Can you work these out from the model? Positions are in its coordinate system, mm. Face numbers are marked on the shaded views. A direction names the side the tool comes from. Round coordinates to 2 decimals unless told otherwise and drop trailing zeros. Order: outer loops, then holes, each group sorted by start corner. A loop starts at its lowest first (then second) coordinate and runs counter-clockwise, first axis right, second up. Notation, with made-up numbers: M 37.5,-9.5 L 62.5,-9.5 A14 cw 62.5,1.5 Z; hole C 81,-36 d1. An arc over 180 degrees is marked long. Answer as a JSON object with one key per item and string values. Group by question number.
from build123d import *

# Parameters (mm, degrees)
BASE_EXTRUSION_DEPTH    = 11
ESQUISSE2_R             = 4
ENL_V_MAT_EXTRU_1_DEPTH = 79.487260113
CHANFREIN1_SIZE         = 0.5
ESQUISSE3_R             = 4
ENL_V_MAT_EXTRU_3_DEPTH = 76.099025835
CHANFREIN2_SIZE         = 0.5
ESQUISSE4_R             = 2
ENL_V_MAT_EXTRU_4_DEPTH = 21.849235277


with BuildPart() as part:
    # Esquisse1 → Base-Extrusion (new body)
    with BuildSketch(Plane.XY):
        with BuildLine():
            Line((23.059250232, 31.5), (52.331191161, 31.5))
            Line((52.331191161, 31.5), (63, 20.831191161))
            Line((63, 20.831191161), (63, 16.5))
            Line((63, 16.5), (25, 16.5))
            Line((25, 16.5), (25, 8.5))
            Line((25, 8.5), (23.059250232, 8.5))
            ThreePointArc((23.059250232, 8.5), (11.332267447, 10.043886573), (0.40445916, 14.570332972))
            Line((0.40445916, 14.570332972), (-15.998711306, 24.040707856))
            ThreePointArc((-15.998711306, 24.040707856), (-20.208003449, 39.75), (-4.498711306, 43.959292144))
            Line((-4.498711306, 43.959292144), (11.90445916, 34.488917259))
            ThreePointArc((11.90445916, 34.488917259), (17.285105485, 32.260180577), (23.059250232, 31.5))
        make_face()
    extrude(amount=BASE_EXTRUSION_DEPTH)

    # Esquisse2 → Enlèv. mat.-Extru.1 (cut, through all)
    with BuildSketch(Plane.XY.offset(11)):
        with Locations((-10.248711306, 34)):
            Circle(ESQUISSE2_R)
    extrude(amount=-ENL_V_MAT_EXTRU_1_DEPTH, mode=Mode.SUBTRACT)

    # Chanfrein1
    chanfrein1_edges = [part.edges().sort_by_distance(p)[0] for p in [
        (-14.248711306, 34, 0),
        (-14.248711306, 34, 11),
    ]]
    chamfer(chanfrein1_edges, length=CHANFREIN1_SIZE)

    # Esquisse3 → Enlèv. mat.-Extru.3 (cut, through all)
    with BuildSketch(Plane(origin=(23.483322458, -13.431543362, 11), x_dir=(1, 0, 0), z_dir=(0, 0, 1))):
        with Locations((-9.483322458, 33.431543362)):
            Circle(ESQUISSE3_R)
    extrude(amount=-ENL_V_MAT_EXTRU_3_DEPTH, mode=Mode.SUBTRACT)

    # Chanfrein2
    chanfrein2_edges = [part.edges().sort_by_distance(p)[0] for p in [
        (10, 20, 0),
        (10, 20, 11),
    ]]
    chamfer(chanfrein2_edges, length=CHANFREIN2_SIZE)

    # Esquisse4 → Enlèv. mat.-Extru.4 (cut)
    with BuildSketch(Plane.XZ.offset(-16.5)):
        with Locations(Location((35, 5.5, 0), (0, 0, 270))):
            Circle(ESQUISSE4_R)
        with Locations(Location((53, 5.5, 0), (0, 0, 270))):
            Circle(ESQUISSE4_R)
    extrude(amount=-ENL_V_MAT_EXTRU_4_DEPTH, mode=Mode.SUBTRACT)


solid = part.part
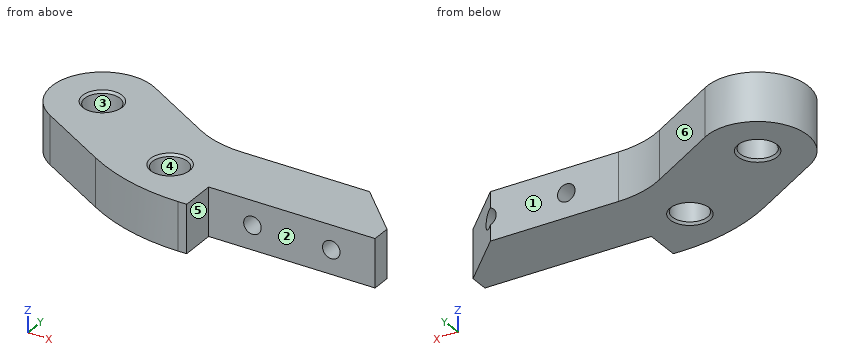
Item 1: Suppose I cut it at C-C, the plane z = 5.5. Write out the boundary of the cut face in (x, y), and give its area (3 significant figures).
Item 2: I need wall thicknesses on line 1 (X direction, y = 18, z = 5.5); line 2 (X direction, y = 21.5, z = 8.25); line 3 (X direction, y = 22.75, z = 5.5). Which ranges of each line are inside material? Lowest first, please.
Item 3: If we mould it in two halves opening along Y, with no side actions, what happens to the marked faces 4, 5 and 6? For each: +Y half, -Y half, draft (parallel to the pull), parting line (faces both ways), or undercut.
Item 4: Suppose I cut it at B-B, the plane x = 35. Write out the boundary of the cut face in (y, z), and give its area (3 significant figures).
Item 5: Suppose I cut it at A-A, the plane y = 20. Write out the boundary of the cut face in (x, z).
Item 6: Suppose I cut it at D-D, the plane z = 1.75. Write out the boundary of the cut face in (x, y), and give its area (3 significant figures).
Item 7: I'm going to push flat-ended pins straight in: pin 1 Ø1.5 at (x, z) = (-8.5, 4.5) entering from -Y; pin 2 Ø5.5 at (x, z) = (38, 5.5) entering from +Y; pin 3 Ø5.5 at (x, z) = (40.5, 3) entering from -Y. Where does each tip first touch, or does it pass through?
Item 8: On a 3-axis mill with a long thin cutter (end or side, diameter ignored), from which of +Z, -Z, +X, -X, +Y, -Y can I reach the whole of each face in a straight line? I mean the marked faces 1, 2 and 3. Say none if no direction works.
Computed:
{
 "1": {"outline": "M -16,24.04 L 0.4,14.57 A45.31 ccw 23.06,8.5 L 25,8.5 L 25,16.5 L 33,16.5 L 33,31.5 L 23.06,31.5 A22.31 cw 11.9,34.49 L -4.5,43.96 A11.5 ccw Z; M 37,16.5 L 51,16.5 L 51,31.5 L 37,31.5 Z; M 55,16.5 L 63,16.5 L 63,20.83 L 55,28.83 Z; hole C -10.25,34 d8; hole C 14,20 d8", "area": "1,390 mm^2"},
 "2": {"line 1": "x = -5.54 to 10.54, 17.46 to 33, 37 to 51, 55 to 63", "line 2": "x = -11.6 to 10.29, 17.71 to 62.33", "line 3": "x = -13.76 to 11.1, 16.9 to 33, 37 to 51, 55 to 61.08"},
 "3": {"face 4": "undercut", "face 5": "draft", "face 6": "+Y half"},
 "4": {"outline": "M 16.5,0 L 31.5,0 L 31.5,3.5 L 16.5,3.5 Z; M 16.5,7.5 L 31.5,7.5 L 31.5,11 L 16.5,11 Z", "area": "105 mm^2"},
 "5": {"outline": "M -9,0 L 9.5,0 L 10,0.5 L 10,10.5 L 9.5,11 L -9,11 Z; M 18,0.5 L 18.5,0 L 63,0 L 63,11 L 18.5,11 L 18,10.5 Z; hole C 35,5.5 d4; hole C 53,5.5 d4"},
 "6": {"outline": "M -16,24.04 L 0.4,14.57 A45.31 ccw 23.06,8.5 L 25,8.5 L 25,16.5 L 63,16.5 L 63,20.83 L 52.33,31.5 L 23.06,31.5 A22.31 cw 11.9,34.49 L -4.5,43.96 A11.5 ccw Z; hole C -10.25,34 d8; hole C 14,20 d8", "area": "1,510 mm^2"},
 "7": {"pin 1": "stops at y = 19.28", "pin 2": "stops at y = 31.5", "pin 3": "stops at y = 16.5"},
 "8": {"face 1": "+Z, -Z, +X, +Y", "face 2": "+Z, -Z, +X, -Y", "face 3": "+Z, -Z"}
}
